Read the model definition and answer for the solid it produces. Units are mm, in the model's axes. Face numbers are marked on the shaded views. A direction names the side the tool comes from. Coordinates: 2 decimals unless noted, no trailing zeros. Loops run counter-clockwise (first coordinate to the right, second up) from the corner with the lowest first, then second, coordinate; pieces in that order, holes last.
Q1. Section A-A (z = 44) is taken. Give the vertices of the cut face in (x, y).
Q2. A flat-ended cylindrical pin translates along its axis: P1, Ø1.2, axis at x = 19, y = -15.5, coming from the -Z side. Find the tip coordinate at first contact, or state that the pin passes through.
Q3. Section D-D (x = -68) is taken. Give the vertices of the cut face in (y, z), then the cut area to 3 significant figures.
Q4. Which of the six approach directions +Z, -Z, +X, -X, +Y, -Y give full straight-line access (tool end or side, diameter ignored) to the marked faces 1 and 2?
Q5. Section C-C (z = 24) is taken. Give the vertices of the cut face in (x, y).
Q6. The mould has two halves that part along X. Classify the marked faces 3, 4, 5 and 6: pulls with the +X half, pulls with the -X half, needs draft (parallel to the pull), parting line crosses it, or undercut.
Q7. Straight lines are drawn through the part: line 1 (Y direction, x = -46.5, z = 42); line 2 (X direction, y = -13, z = 24); line 3 (Z direction, x = 7.5, y = -20.5). For each, find the intervals that lie inside material, in ascending order.
Q8. Section B-B (y = -41) is taken. Give the vertices of the cut face in (x, z), then the cut area to 3 significant figures.
from build123d import *

# Parameters (mm, degrees)
ESQUISSE1_W                  = 109
ESQUISSE1_H                  = 59
BOSS_EXTRU_1_DEPTH           = 50
ESQUISSE2_W                  = 101
ESQUISSE2_H                  = 51
ENL_V_MAT_EXTRU_1_DEPTH      = 47
ENL_V_MAT_EXTRU_2_DEPTH      = 118.384292451
ENL_V_MAT_EXTRU_2_DEPTH_BACK = 21
ESQUISSE3_W                  = 7
ESQUISSE3_H                  = 9.559529104
ESQUISSE3_W_2                = 12
ESQUISSE3_H_2                = 16
ESQUISSE4_R                  = 24
ENL_V_MAT_EXTRU_3_DEPTH      = 73


with BuildPart() as part:
    # Esquisse1 → Boss.-Extru.1 (new body)
    with BuildSketch(Plane.XY):
        with Locations((-33.806693485, -29.5)):
            Rectangle(ESQUISSE1_W, ESQUISSE1_H)
    extrude(amount=BOSS_EXTRU_1_DEPTH)

    # Esquisse2 → Enlèv. mat.-Extru.1 (cut)
    with BuildSketch(Plane.XY):
        with Locations((-33.806693485, -29.5)):
            Rectangle(ESQUISSE2_W, ESQUISSE2_H)
    extrude(amount=ENL_V_MAT_EXTRU_1_DEPTH, mode=Mode.SUBTRACT)

    # Esquisse3 → Enlèv. mat.-Extru.2 (cut, two sides: drawn at the far end of the back side and taken through both)
    with BuildSketch(Plane(origin=(0, 0, 0), x_dir=(0, 0, -1), z_dir=(1, 0, 0)).offset(-ENL_V_MAT_EXTRU_2_DEPTH_BACK)):
        with Locations((-24.5, -40.983092888)):
            Rectangle(ESQUISSE3_W, ESQUISSE3_H)
        with Locations((-6, -18)):
            Rectangle(ESQUISSE3_W_2, ESQUISSE3_H_2)
    extrude(amount=ENL_V_MAT_EXTRU_2_DEPTH + ENL_V_MAT_EXTRU_2_DEPTH_BACK, mode=Mode.SUBTRACT)

    # Esquisse4 → Enlèv. mat.-Extru.3 (cut)
    with BuildSketch(Plane.XY):
        with Locations(Location((-56.773597779, -29.250359736, 0), (0, 0, 180))):
            Circle(ESQUISSE4_R)
    extrude(amount=ENL_V_MAT_EXTRU_3_DEPTH, mode=Mode.SUBTRACT)


solid = part.part
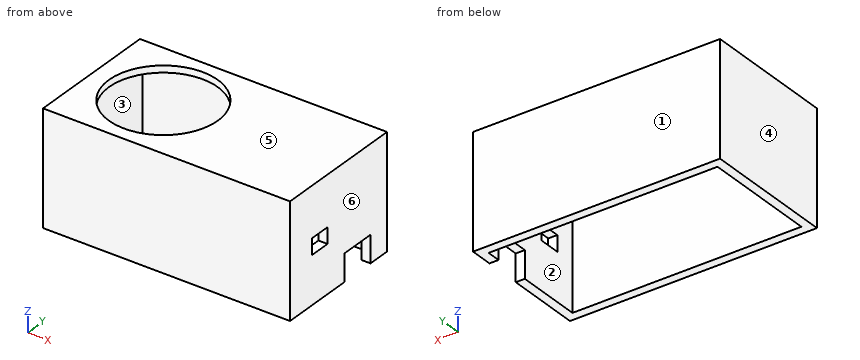
Numbers:
1. outline: (-88.31, -59) - (20.69, -59) - (20.69, 0) - (-88.31, 0) - close; hole (-84.31, -55) - (16.69, -55) - (16.69, -4) - (-84.31, -4) - close
2. P1: stops at z = 12
3. outline: (-59, 0) - (-55, 0) - (-55, 47) - (-50.46, 47) - (-50.46, 50) - (-59, 50) - close; (-8.04, 47) - (-4, 47) - (-4, 0) - (0, 0) - (0, 50) - (-8.04, 50) - close
3. area: 426 mm2
4. face 1: +Z, -Z, +X, -X, +Y
4. face 2: -Z
5. outline: (-88.31, -59) - (20.69, -59) - (20.69, -45.76) - (16.69, -45.76) - (16.69, -55) - (-84.31, -55) - (-84.31, -4) - (16.69, -4) - (16.69, -36.2) - (20.69, -36.2) - (20.69, 0) - (-88.31, 0) - close
6. face 3: undercut
6. face 4: pulls with the -X half
6. face 5: needs draft
6. face 6: pulls with the +X half
7. line 1: y = -59 to -55, -4 to 0
7. line 2: x = -88.31 to -84.31, 16.69 to 20.69
7. line 3: z = 47 to 50
8. outline: (-88.31, 0) - (-84.31, 0) - (-84.31, 47) - (-77.7, 47) - (-77.7, 50) - (-88.31, 50) - close; (-35.85, 47) - (16.69, 47) - (16.69, 28) - (20.69, 28) - (20.69, 50) - (-35.85, 50) - close; (16.69, 0) - (20.69, 0) - (20.69, 21) - (16.69, 21) - close
8. area: 549 mm2
